Could you check a few things on this model? Use its own coordinates, in mm. Face numbers are marked on the shaded views. Give positions to 0.01 mm unless a question says otherwise; leave off trailing zeros. Loops run counter-clockwise (first coordinate to the right, second up) from the corner with the lowest first, then second, coordinate; pieces in that order, holes last. Notation, with made-up numbers: M 24.5,86.25 L 77.5,86.25 A27 cw 77.5,112.25 Z; hole C -11.5,84.5 d8. An arc over 180 degrees is marked long. Return JSON: item names as keys, results as strings. Group by question number.
1. For pin 1 (5 mm diameter, centred on y = 971, z = 38.5, fed in from -X); pin 2 (1 mm diameter, centred on y = 280.5, z = 42, fed in from +X); pin 3 (1.5 mm diameter, centred on x = -13, z = 27.5, fed in from -Y), each with a flat end and sliding along its axis, tell me the tip position at first contact or that it passes through.
2. Please list where these lines run through material, in increasing order: line 1 (Y direction, x = 0.5, z = 0); line 2 (Z direction, x = 20.5, y = 596); line 3 (X direction, y = 703, z = 40).
3. If we section it at B-B (z = 0): Write out the boundary of the cut face in (x, y), plus the area to 3 significant figures.
4. If we section it at A-A (x = 20): Write out the boundary of the cut face in (y, z).
5. If we section it at C-C (y = 900): Write out the boundary of the cut face in (x, z), plus the area to 3 significant figures.
6. If we mould it in two halves opening along Z, with no side actions, what happens to the marked faces 1, 2, 3 and 4? For each: +Z half, -Z half, draft (parallel to the pull), parting line (faces both ways), or undercut.
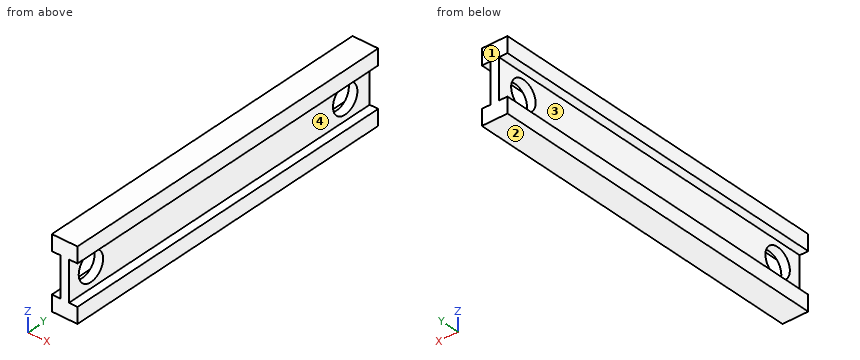
```python
from build123d import *

# Parameters (mm, degrees)
BOSS_EXTRUDE1_DEPTH = 1230
SKETCH2_R           = 50
CUT_EXTRUDE1_DEPTH  = 1200
SKETCH3_R           = 50
CUT_EXTRUDE2_DEPTH  = 1200
SCALE1_SCALE        = 0.75


with BuildPart() as part:
    # Sketch1 → Boss-Extrude1 (new body)
    with BuildSketch(Plane(origin=(0, 0, 0), x_dir=(1, 0, 0), z_dir=(0, 1, 0))):
        Polygon((-45, -70), (-45, -125), (45, -125), (45, -70), (15, -70), (15, 70), (45, 70), (45, 125), (-45, 125), (-45, 70), (-15, 70), (-15, -70), align=None)
    extrude(amount=BOSS_EXTRUDE1_DEPTH)

    # Sketch2 → Cut-Extrude1 (cut)
    with BuildSketch(Plane(origin=(15, 0, 0), x_dir=(0, 0, -1), z_dir=(1, 0, 0))):
        with Locations((0, 90)):
            Circle(SKETCH2_R)
    extrude(amount=-CUT_EXTRUDE1_DEPTH, mode=Mode.SUBTRACT)

    # Sketch3 → Cut-Extrude2 (cut)
    with BuildSketch(Plane(origin=(15, 0, 0), x_dir=(0, 0, -1), z_dir=(1, 0, 0))):
        with Locations((0, 1130)):
            Circle(SKETCH3_R)
    extrude(amount=-CUT_EXTRUDE2_DEPTH, mode=Mode.SUBTRACT)


with BuildPart() as part_1:
    # Scale1: scaled about (0, 615.139653144, 0)
    add(part.part.scale(SCALE1_SCALE).moved(Location((0, 153.784913286, 0))))


solid = part_1.part
```
Answer:
{
 "1": {"pin 1": "stops at x = -11.25", "pin 2": "stops at x = 11.25", "pin 3": "passes through"},
 "2": {"line 1": "y = 153.78 to 183.78, 258.78 to 963.78, 1038.78 to 1076.28", "line 2": "z = -93.75 to -52.5, 52.5 to 93.75", "line 3": "x = -11.25 to 11.25"},
 "3": {"outline": "M -11.25,153.78 L 11.25,153.78 L 11.25,183.78 L -11.25,183.78 Z; M -11.25,258.78 L 11.25,258.78 L 11.25,963.78 L -11.25,963.78 Z; M -11.25,1038.78 L 11.25,1038.78 L 11.25,1076.28 L -11.25,1076.28 Z", "area": "17,400 mm²"},
 "4": {"outline": "M 153.78,-93.75 L 1076.28,-93.75 L 1076.28,-52.5 L 153.78,-52.5 Z; M 153.78,52.5 L 1076.28,52.5 L 1076.28,93.75 L 153.78,93.75 Z"},
 "5": {"outline": "M -33.75,-93.75 L 33.75,-93.75 L 33.75,-52.5 L 11.25,-52.5 L 11.25,52.5 L 33.75,52.5 L 33.75,93.75 L -33.75,93.75 L -33.75,52.5 L -11.25,52.5 L -11.25,-52.5 L -33.75,-52.5 Z", "area": "7,930 mm²"},
 "6": {"face 1": "draft", "face 2": "-Z half", "face 3": "undercut", "face 4": "undercut"}
}
